Study the drawing (mm; zero at the part's minimum x, y, z) and answer. A direction names the side the tool comes from. Coordinates: 2 decimals unless noted, no trailing zeros. Write each loop counter-clockwise with the first axis right and the second up, starting at its lowest first coordinate (ties: lowest second). Pieces come first, ordered by that corner, then holes. Notation, with made-up numbers: (5.5, -27.5) -> (47.5, -27.5) arc R18 cw to (47.5, -17.5) -> close; hole circle Ø2 at (16, 75). An arc over 180 degrees is marked (long way). Answer in a Markdown table with one row per item. Add a question column.
Item 1: Which of the six approach directions +Z, -Z, +X, -X, +Y, -Y give full straight-line access (tool end or side, diameter ignored) to the marked faces 1, 2 and 3?
Item 2: Given pin 1 Ø4 at (y, z) = (7, 13) entering from +X; pin 2 Ø1 at (x, z) = (30, 14) entering from +Y; pin 3 Ø6.5 at (y, z) = (5.5, 7) entering from -X, each flat-ended and moving along its own axis, determine where each tip first touches the part or whether it passes through.
Item 3: Straight lines are drawn through the part: line 1 (Y direction, x = 13, z = 15) (1 decimal); line 2 (Z direction, x = 39, y = 30); line 3 (X direction, y = 3, z = 7). For each, find the intervals that lie inside material, in ascending order. Write a range as from..to.
Item 4: Section D-D on y = 25 is taken. Write down the section's boundary in (x, z), then the cut area to 3 significant figures.
Item 5: Section A-A on y = 3 is taken. Write down the section's boundary in (x, z), then the cut area to 3 significant figures.
Item 6: Section C-C on z = 5.5 is taken. Write down the section's boundary in (x, y) (1 decimal).
Item 7: Section B-B on x = 50.5 is taken. Write down the section's boundary in (y, z) (1 decimal).
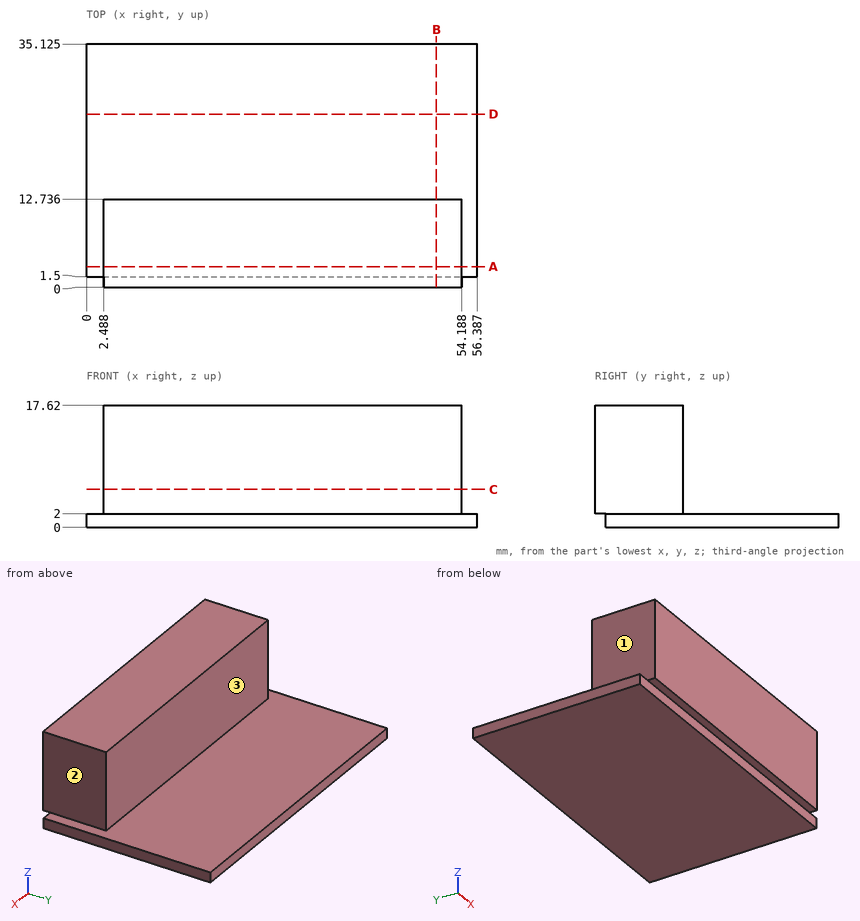
Results below:
| question | item | result |
|---|---|---|
| 1 | face 1 | +Z, -X, +Y, -Y |
| 1 | face 2 | +Z, +X, +Y, -Y |
| 1 | face 3 | +Z, +X, -X, +Y |
| 2 | pin 1 | stops at x = 54.19 |
| 2 | pin 2 | stops at y = 12.74 |
| 2 | pin 3 | stops at x = 2.49 |
| 3 | line 1 | y = 0..12.7 |
| 3 | line 2 | z = 0..2 |
| 3 | line 3 | x = 2.49..54.19 |
| 4 | outline | (0, 0) -> (56.39, 0) -> (56.39, 2) -> (0, 2) -> close |
| 4 | area | 113 mm2 |
| 5 | outline | (0, 0) -> (56.39, 0) -> (56.39, 2) -> (54.19, 2) -> (54.19, 17.62) -> (2.49, 17.62) -> (2.49, 2) -> (0, 2) -> close |
| 5 | area | 920 mm2 |
| 6 | outline | (2.5, 0) -> (54.2, 0) -> (54.2, 12.7) -> (2.5, 12.7) -> close |
| 7 | outline | (0, 2) -> (1.5, 2) -> (1.5, 0) -> (35.1, 0) -> (35.1, 2) -> (12.7, 2) -> (12.7, 17.6) -> (0, 17.6) -> close |
